The listing builds one solid part. Answer for the finished solid, in the listing's coordinates (mm). Coordinates: 2 decimals unless noted, no trailing zeros. Order: outer loops, then holes, each group sorted by start corner. A loop starts at its lowest first (then second) coordinate and runs counter-clockwise, first axis right, second up.
```python
from build123d import *

# Parameters (mm, degrees)
F0_W     = 127
F0_H     = 12.7
F1_DEPTH = 1016
F2_DEPTH = 533.4


with BuildPart() as f1:
    # F0 (on Front) → F1 (new body)
    with BuildSketch(Plane.XZ):
        with Locations((-685.8, 6.35)):
            Rectangle(F0_W, F0_H)
        Polygon((-622.3, 0), (0, 0), (622.3, 0), (622.3, 12.7), (-622.3, 12.7), align=None)
        with Locations((685.8, 6.35)):
            Rectangle(F0_W, F0_H)
    extrude(amount=F1_DEPTH)

    # F0 (on Front) → F2 (cut)
    with BuildSketch(Plane.XZ):
        with Locations((-685.8, 6.35)):
            Rectangle(F0_W, F0_H)
        with Locations((685.8, 6.35)):
            Rectangle(F0_W, F0_H)
    extrude(amount=F2_DEPTH, mode=Mode.SUBTRACT)


solid = f1.part
```
(1) Each of these flat-tipped pins is pushed along its axis until it touches: pin 1 Ø4 at (x, z) = (711.5, 7.5) entering from +Y; pin 2 Ø3 at (y, z) = (-286.5, 7) entering from +X; pin 3 Ø6 at (x, z) = (-279.5, 9) entering from +Y; pin 4 Ø2 at (y, z) = (-203, 3.5) entering from -X. Where does it stop, or does it pass through?
(2) Find section B-B (y = -307.5). Write down the section's boundary in (x, z), and give its area (3 significant figures).
(3) Find section A-A (z = 3.5). Write down the section's boundary in (x, y).
(4) Consider line 1 (X direction, y = -70.5, z = 11.5). Determine where the line is inside the solid, lowest interval first.
Findings below:
1. pin 1: stops at y = -533.4
1. pin 2: stops at x = 622.3
1. pin 3: stops at y = 0
1. pin 4: stops at x = -622.3
2. outline: (-622.3, 0) - (622.3, 0) - (622.3, 12.7) - (-622.3, 12.7) - close
2. area: 15,800 mm2
3. outline: (-749.3, -1016) - (749.3, -1016) - (749.3, -533.4) - (622.3, -533.4) - (622.3, 0) - (-622.3, 0) - (-622.3, -533.4) - (-749.3, -533.4) - close
4. line 1: x = -622.3 to 622.3
